Autodesk Inventor part; units mm, degrees
ref_plane "YZ Plane" through (0, 0, 0) normal (1, 0, 0) x (0, 1, 0)
ref_plane "XZ Plane" through (0, 0, 0) normal (0, 1, 0) x (-1, 0, 0)
ref_plane "XY Plane" through (0, 0, 0) normal (0, 0, 1) x (1, 0, 0)
sketch "Sketch1" plane through (0, 0, 0) normal (0, 0, 1) x (1, 0, 0)
  line L0 (-8.0405, 16.8694) -> (12.9595, 16.8694)
  line L1 (12.9595, 16.8694) -> (12.9595, -34.1306)
  line L2 (12.9595, -34.1306) -> (-8.0405, -34.1306)
  line L3 (-8.0405, -34.1306) -> (-8.0405, 16.8694)
  circle A0 centre (-3.2405, 14.8694) radius 1.05
  circle A1 centre (8.1595, 14.8694) radius 1.05
  circle A2 centre (-3.2405, -32.1306) radius 1.05
  circle A3 centre (8.1595, -32.1306) radius 1.05
  circle A4 centre (-3.2405, 14.8694) radius 1.15
  circle A5 centre (8.1595, 14.8694) radius 1.15
  circle A6 centre (-3.2405, -32.1306) radius 1.15
  circle A7 centre (8.1595, -32.1306) radius 1.15
  point P0 (0, 0)
  dimension "d0" = 21
  dimension "d1" = 51
  dimension "d2" = 2.1
  dimension "d3" = 2.1
  dimension "d4" = 2.1
  dimension "d5" = 2.1
  dimension "d6" = 2
  dimension "d7" = 2
  dimension "d8" = 2
  dimension "d9" = 2
  dimension "d10" = 11.4
  dimension "d11" = 4.8
  dimension "d12" = 11.4
  dimension "d13" = 4.8
  dimension "d14" = 0.1
  dimension "d15" = 0.1
  dimension "d16" = 0.1
  dimension "d17" = 0.1
extrude "Extrusion1" add sketch "Sketch1" along normal blind 2.54 contours L0 L1 L2 L3
properties part number "PicoTest"
Check sheet for the modelled part. Datum: model origin and axes. Units: mm. Round coordinates to 2 decimals unless told otherwise and drop trailing zeros. Loops run counter-clockwise (first coordinate to the right, second up) from the corner with the lowest first, then second, coordinate; pieces in that order, holes last.
1. Mould release check, pull along Y, two halves, no side actions. Record for faces 1 (the flat face through (-8.04, -9, 1)), 2 (the flat face through (2, 16.869, 1)), 3 (the cylindrical face through (7.25, 15.57, 1.25)): released by +Y, released by -Y, zero draft, split by the parting line, or undercut.
2. Scan lines: probe 1 along Y at (x, z) = (7.25, 0.65); probe 2 along X at (y, z) = (14, 0.45); probe 3 along Y at (x, z) = (7.5, 1.8). Record each from-to range of solid material in increasing order.
3. Sectioned sample at A-A on z = 1. Record the boundary of the cut face in (x, y).
4. Gauge pin test, flat end, axial feed: pin 1 Ø1.8 at (x, y) = (8.16, 14.87) entering from -Z. Record the tip position at first contact, or that the pin passes through.
Recorded:
1. face 1: zero draft
1. face 2: released by +Y
1. face 3: undercut
2. probe 1: y = -34.13 to -32.83, -31.43 to 14.17, 15.57 to 16.87
2. probe 2: x = -8.04 to -3.99, -2.49 to 7.41, 8.91 to 12.96
2. probe 3: y = -34.13 to -33.07, -31.19 to 13.93, 15.81 to 16.87
3. outline: (-8.04, -34.13) - (12.96, -34.13) - (12.96, 16.87) - (-8.04, 16.87) - close; hole circle Ø2.3 at (-3.24, -32.13); hole circle Ø2.3 at (-3.24, 14.87); hole circle Ø2.3 at (8.16, -32.13); hole circle Ø2.3 at (8.16, 14.87)
4. pin 1: passes through
